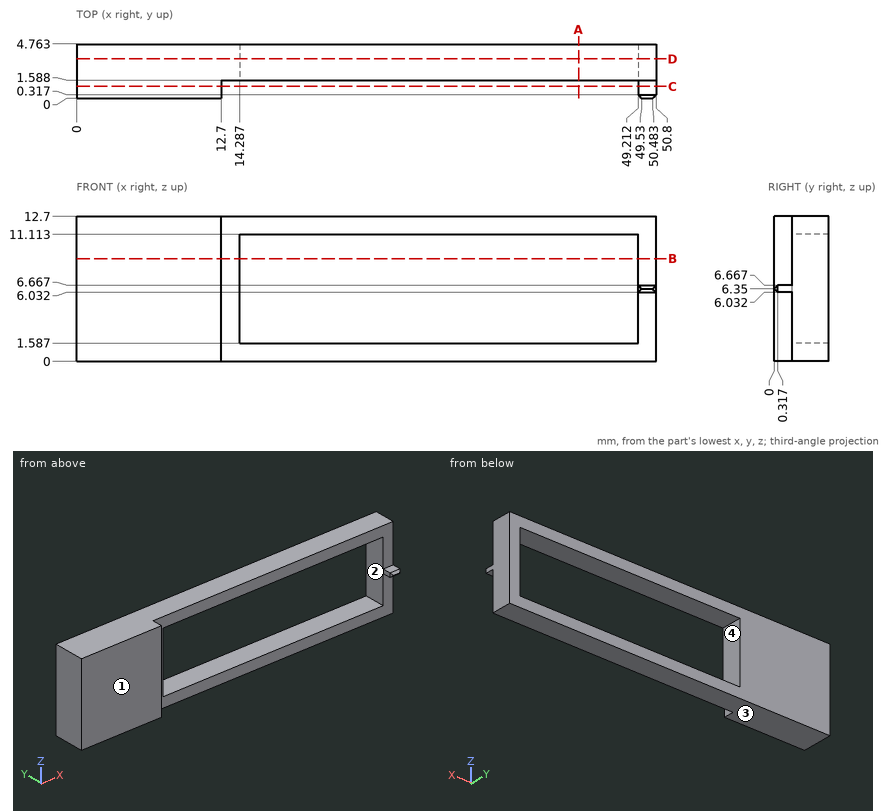
Study the drawing (mm; zero at the part's minimum x, y, z) and answer. Round coordinates to 2 decimals unless told otherwise and drop trailing zeros. Write each loop counter-clockwise with the first axis right and the second up, starting at its lowest first coordinate (ties: lowest second). Pieces come first, ordered by that corner, then holes.
1) Flat-ended cylindrical pins translate along their axes: P1, Ø1, axis at x = 50, y = 0.5, coming from the -Z side; P2, Ø0.6, axis at x = 49.5, y = 1, coming from the +Z side. Find the tip coordinate at first contact, or state that the pin passes through.
2) A cutting plane is placed at C-C on y = 1.05. Determine the outline of the cut face in (x, z), and give its area (3 significant figures).
3) A cutting plane is placed at A-A on x = 44. Determine the outline of the cut face in (y, z), and give its area (3 significant figures).
4) Determine the mould class of the marked faces 1, 2, 3 and 4 for opening direction Z: pulls with the +Z half, pulls with the -Z half, needs draft (parallel to the pull), parting line crosses it, or undercut.
5) A cutting plane is placed at B-B on z = 9. Determine the outline of the cut face in (x, y).
6) A cutting plane is placed at D-D on y = 3.45. Determine the outline of the cut face in (x, z).
7) Consider probe 1 along X at (y, z) = (4.55, 7.5); probe 2 along X at (y, z) = (0.9, 6.25); probe 3 along Z at (x, y) = (15.5, 2.1). Determine where each line is inside the solid, lowest interval first.
Entries:
1. P1: stops at z = 6.03
1. P2: stops at z = 6.67
2. outline: (0, 0) - (12.7, 0) - (12.7, 12.7) - (0, 12.7) - close; (49.21, 6.03) - (50.8, 6.03) - (50.8, 6.67) - (49.21, 6.67) - close
2. area: 162 mm2
3. outline: (1.59, 0) - (4.76, 0) - (4.76, 1.59) - (1.59, 1.59) - close; (1.59, 11.11) - (4.76, 11.11) - (4.76, 12.7) - (1.59, 12.7) - close
3. area: 10.1 mm2
4. face 1: needs draft
4. face 2: undercut
4. face 3: pulls with the -Z half
4. face 4: undercut
5. outline: (0, 0) - (12.7, 0) - (12.7, 1.59) - (14.29, 1.59) - (14.29, 4.76) - (0, 4.76) - close; (49.21, 1.59) - (50.8, 1.59) - (50.8, 4.76) - (49.21, 4.76) - close
6. outline: (0, 0) - (50.8, 0) - (50.8, 12.7) - (0, 12.7) - close; hole (14.29, 1.59) - (49.21, 1.59) - (49.21, 11.11) - (14.29, 11.11) - close
7. probe 1: x = 0 to 14.29, 49.21 to 50.8
7. probe 2: x = 0 to 12.7, 49.21 to 50.8
7. probe 3: z = 0 to 1.59, 11.11 to 12.7
